Model file for the job. Use its own axes, mm. Face numbers are marked on the shaded views. A direction names the side the tool comes from. Round coordinates to 2 decimals unless told otherwise and drop trailing zeros. Loops run counter-clockwise (first coordinate to the right, second up) from the corner with the lowest first, then second, coordinate; pieces in that order, holes last. Notation, with made-up numbers: (24.5, 57.25) -> (50.5, 57.25) arc R29 cw to (50.5, 77.25) -> close; hole circle Ø10 at (-34.75, -12.5). An arc over 180 degrees is marked (long way). Use a Markdown table: item, result.
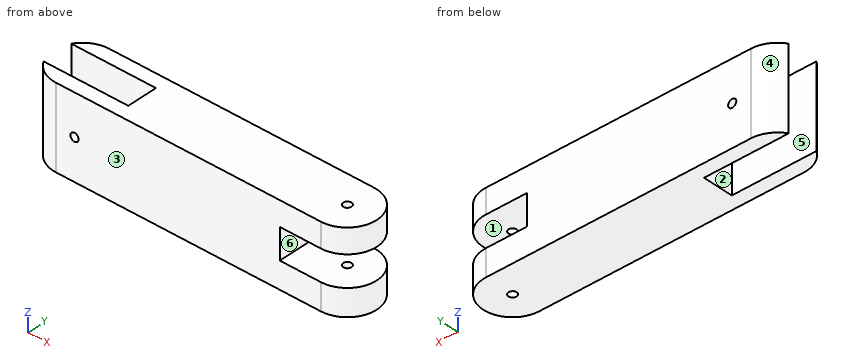
from build123d import *

# Parameters (mm, degrees)
RESSALTO_EXTRUS_O1_DEPTH = 40
ESBO_O2_R                = 2
CORTE_EXTRUS_O1_DEPTH    = 40
ESBO_O3_W                = 45.5934118
ESBO_O3_H                = 15
CORTE_EXTRUS_O2_DEPTH    = 40
ESBO_O4_R                = 2
CORTE_EXTRUS_O3_DEPTH    = 40
ESBO_O6_W                = 60.91322231
ESBO_O6_H                = 15
CORTE_EXTRUS_O5_DEPTH    = 62.5


with BuildPart() as part:
    # Esboço1 → Ressalto-extrusão1 (new body)
    with BuildSketch(Plane.XY):
        with BuildLine():
            Line((-56.556913458, 14.405805893), (73.443086542, 14.405805893))
            ThreePointArc((73.443086542, 14.405805893), (87.848892435, 0), (73.443086542, -14.405805893))
            Line((73.443086542, -14.405805893), (-56.556913458, -14.405805893))
            ThreePointArc((-56.556913458, -14.405805893), (-70.96271935, 0), (-56.556913458, 14.405805893))
        make_face()
    extrude(amount=RESSALTO_EXTRUS_O1_DEPTH)

    # Esboço2 → Corte-extrusão1 (cut, symmetric)
    with BuildSketch(Plane.XY.offset(40)):
        with Locations((73.443086542, 0)):
            Circle(ESBO_O2_R)
    extrude(amount=CORTE_EXTRUS_O1_DEPTH, both=True, mode=Mode.SUBTRACT)

    # Esboço3 → Corte-extrusão2 (cut, symmetric)
    with BuildSketch(Plane.XY.offset(40)):
        with Locations((-50.120588086, 0)):
            Rectangle(ESBO_O3_W, ESBO_O3_H)
    extrude(amount=CORTE_EXTRUS_O2_DEPTH, both=True, mode=Mode.SUBTRACT)

    # Esboço4 → Corte-extrusão3 (cut, symmetric)
    with BuildSketch(Plane(origin=(0, 14.405805893, 0), x_dir=(1, 0, 0), z_dir=(0, 1, 0))):
        with Locations(Location((-47.413412599, -20, 0), (0, 0, 270))):
            Circle(ESBO_O4_R)
    extrude(amount=CORTE_EXTRUS_O3_DEPTH, both=True, mode=Mode.SUBTRACT)

    # Esboço6 → Corte-extrusão5 (cut, symmetric)
    with BuildSketch(Plane(origin=(0, 14.405805893, 0), x_dir=(1, 0, 0), z_dir=(0, 1, 0))):
        with Locations((83.774809185, -20.540511229)):
            Rectangle(ESBO_O6_W, ESBO_O6_H)
    extrude(amount=CORTE_EXTRUS_O5_DEPTH, both=True, mode=Mode.SUBTRACT)


solid = part.part
Q1. Band-saw the part on B-B, the plane z = 20. Give the cut face in (x, y), plus the area to 3 significant figures.
Results list:
| item | result |
|---|---|
| outline | (-68.86, -7.5) arc R14.41 ccw to (-56.56, -14.41) -> (-49.41, -14.41) -> (-49.41, -7.5) -> close; (-68.86, 7.5) -> (-49.41, 7.5) -> (-49.41, 14.41) -> (-56.56, 14.41) arc R14.41 ccw to start; (-45.41, -14.41) -> (53.32, -14.41) -> (53.32, 14.41) -> (-45.41, 14.41) -> (-45.41, 7.5) -> (-27.32, 7.5) -> (-27.32, -7.5) -> (-45.41, -7.5) -> close |
| area | 2,790 mm² |
Q2. Tool access for the marked faces 1, 2 and 3: list every direction of +Z, -Z, +X, -X, +Y, -Y with a clear straight run to the whole face (end or side of a thin tool).
Results list:
| item | result |
|---|---|
| face 1 | +X, +Y, -Y |
| face 2 | +Z, -Z, -X |
| face 3 | +Z, -Z, +X, -X, -Y |
Q3. Flat gauge pins, fed straight in: pin 1 (12 mm diameter, centred on y = 2.5, z = 19.5, fed in from +X); pin 2 (3.5 mm diameter, centred on x = -47.41, z = 20, fed in from -Y); pin 3 (1 mm diameter, centred on y = -2, z = 8, fed in from -X); pin 4 (5 mm diameter, centred on y = -11.5, z = 8, fed in from -X). Where does each tip first touch, or does it go through?
Results list:
| item | result |
|---|---|
| pin 1 | stops at x = 53.32 |
| pin 2 | passes through |
| pin 3 | stops at x = -27.32 |
| pin 4 | stops at x = -67.81 |
Q4. Band-saw the part on A-A, the plane x = 63. Give the cut face in (y, z).
Results list:
| item | result |
|---|---|
| outline | (-14.41, 0) -> (14.41, 0) -> (14.41, 13.04) -> (-14.41, 13.04) -> close; (-14.41, 28.04) -> (14.41, 28.04) -> (14.41, 40) -> (-14.41, 40) -> close |
Q5. Band-saw the part on C-C, the plane y = 0. Give the cut face in (x, z), plus the area to 3 significant figures.
Results list:
| item | result |
|---|---|
| outline | (-27.32, 0) -> (71.44, 0) -> (71.44, 13.04) -> (53.32, 13.04) -> (53.32, 28.04) -> (71.44, 28.04) -> (71.44, 40) -> (-27.32, 40) -> close; (75.44, 0) -> (87.85, 0) -> (87.85, 13.04) -> (75.44, 13.04) -> close; (75.44, 28.04) -> (87.85, 28.04) -> (87.85, 40) -> (75.44, 40) -> close |
| area | 3,990 mm² |
Q6. Pull direction Y, two halves, no side cores. Call the marked faces 4, 5 and 6: released by +Y, released by -Y, zero draft, split by the parting line, or undercut.
Results list:
| item | result |
|---|---|
| face 4 | released by +Y |
| face 5 | undercut |
| face 6 | zero draft |
Q7. Drill centre lines: L1, parallel to Z at x = 60.5, y = 9; L2, parallel to X at y = -4.25, z = 27.5; L3, parallel to X at y = -11.5, z = 20. Where is each one in solid material? Low to high. Write a range as from..to.
Results list:
| item | result |
|---|---|
| L1 | z = 0..13.04, 28.04..40 |
| L2 | x = -27.32..53.32 |
| L3 | x = -65.23..-49.41, -45.41..53.32 |
Q8. Band-saw the part on D-D, the plane z = 34.5. Give the cut face in (x, y), plus the area to 3 significant figures.
Results list:
| item | result |
|---|---|
| outline | (-68.86, -7.5) arc R14.41 ccw to (-56.56, -14.41) -> (73.44, -14.41) arc R14.41 ccw to (73.44, 14.41) -> (-56.56, 14.41) arc R14.41 ccw to (-68.86, 7.5) -> (-27.32, 7.5) -> (-27.32, -7.5) -> close; hole circle Ø4 at (73.44, 0) |
| area | 3,740 mm² |
